Model file for the job. Use its own axes, mm. Coordinates: 2 decimals unless noted, no trailing zeros. Loops run counter-clockwise (first coordinate to the right, second up) from the corner with the lowest first, then second, coordinate; pieces in that order, holes last. Notation, with made-up numbers: M 35,-11.75 L 49,-11.75 A24 cw 49,21.25 Z; hole C 10,-29.75 d8. An arc over 180 degrees is marked long. Write item = value, one per line. Start each with the question number.
from build123d import *

# Parameters (mm, degrees)
BOSS_EXTRUDE1_DEPTH = 50
CUT_EXTRUDE1_DEPTH  = 105.547835941
SKETCH3_R           = 2.5
CUT_EXTRUDE2_DEPTH  = 105.547835941
SKETCH4_W           = 80
SKETCH4_H           = 10
CUT_EXTRUDE3_DEPTH  = 82.240384046
CUT_EXTRUDE4_START  = -10.5
CUT_EXTRUDE4_DEPTH  = 10.5


# Read off the part's stored shape, not the designer's step: Cut-Extrude4
with BuildPart() as part:
    # Sketch1 → Boss-Extrude1 (new body)
    with BuildSketch(Plane.XY):
        Polygon((29.5, 60), (29.5, 10), (-40, 10), (-40, 0), (40, 0), (40, 60), align=None)
    extrude(amount=-BOSS_EXTRUDE1_DEPTH)

    # Sketch2 → Cut-Extrude1 (cut, through all)
    with BuildSketch(Plane.ZY.offset(-29.5)):
        with BuildLine():
            Line((-50, 60), (-50, 35))
            ThreePointArc((-50, 35), (-42.67766953, 52.67766953), (-25, 60))
            Line((-25, 60), (-50, 60))
        make_face()
        with BuildLine():
            Line((0, 60), (-25, 60))
            ThreePointArc((-25, 60), (-7.32233047, 52.67766953), (0, 35))
            Line((0, 35), (0, 60))
        make_face()
    extrude(amount=-CUT_EXTRUDE1_DEPTH, mode=Mode.SUBTRACT)

    # Sketch3 → Cut-Extrude2 (cut, through all)
    with BuildSketch(Plane.ZY.offset(-29.5)):
        with Locations((-25, 35)):
            Circle(SKETCH3_R)
    extrude(amount=-CUT_EXTRUDE2_DEPTH, mode=Mode.SUBTRACT)

    # Sketch4 → Cut-Extrude3 (cut, through all)
    with BuildSketch(Plane(origin=(0, 10, 0), x_dir=(1, 0, 0), z_dir=(0, 1, 0))):
        with Locations((0, 45)):
            Rectangle(SKETCH4_W, SKETCH4_H)
        with Locations((0, 5)):
            Rectangle(SKETCH4_W, SKETCH4_H)
    extrude(amount=-CUT_EXTRUDE3_DEPTH, mode=Mode.SUBTRACT)

    # Cut-Extrude4 outline → Cut-Extrude4 (cut)
    with BuildSketch(Plane.ZY.offset(-29.5).offset(CUT_EXTRUDE4_START)):
        with BuildLine():
            ThreePointArc((-45, 20), (-48.717082451, 27.09430585), (-50, 35))
            Line((-50, 35), (-50, 10))
            Line((-50, 10), (-40, 10))
            ThreePointArc((-40, 10), (-40.513167019, 13.16227766), (-42, 16))
            Line((-42, 16), (-45, 20))
        make_face()
        with BuildLine():
            ThreePointArc((0, 35), (-1.293142852, 27.063695813), (-5.038793932, 19.948413628))
            Line((-5.038793932, 19.948413628), (-8, 16))
            ThreePointArc((-8, 16), (-9.486832981, 13.16227766), (-10, 10))
            Line((-10, 10), (0, 10))
            Line((0, 10), (0, 35))
        make_face()
    extrude(amount=CUT_EXTRUDE4_DEPTH, mode=Mode.SUBTRACT)


solid = part.part
Item 1: Pin check, flat tips, straight feed: pin 1 Ø1.5 at (x, z) = (-13.5, -41.5) entering from +Y; pin 2 Ø12 at (y, z) = (37.5, -13.5) entering from -X; pin 3 Ø3 at (x, y) = (12, 6.5) entering from +Z; pin 4 Ø8 at (x, z) = (24, -21.5) entering from +Y. Stop position of each tip, or through.
Item 2: Cut at B-B (x = -1). Give the cut face in (y, z), plus the area to 3 significant figures.
Item 3: Probe L1, parallel to Y at x = 33.5, z = -25; L2, parallel to X at y = 29, z = -46.5; L3, parallel to Y at x = -35, z = -30.5. List the from-to ranges inside material, lowest first.
Item 4: Cut at A-A (y = 18.5). Give the cut face in (x, z) (3 decimals), plus the area to 3 significant figures.
Item 5: Pull direction Y, two halves, no side cores. Call faces 1 (the flat face through (-1, 0, -25)), 2 (the cylindrical face through (34.68, 36.69, -26.84)), 3 (the flat face through (-5, 10, -25)), 4 (the flat face through (29.5, 30, -25)): +Y half, -Y half, draft (parallel to the pull), parting line (faces both ways), or undercut.
Reported:
q1.pin_1 = through
q1.pin_2 = 29.5
q1.pin_3 = -10
q1.pin_4 = 10
q2.outline = M 0,-40 L 10,-40 L 10,-10 L 0,-10 Z
q2.area = 300 mm^2
q3.L1 = 0 to 32.5, 37.5 to 60
q3.L2 = 29.5 to 40
q3.L3 = 0 to 10
q4.outline = M 29.5,-43.875 L 40,-43.875 L 40,-6.125 L 29.5,-6.125 Z
q4.area = 396 mm^2
q5.face_1 = -Y half
q5.face_2 = undercut
q5.face_3 = +Y half
q5.face_4 = draft
